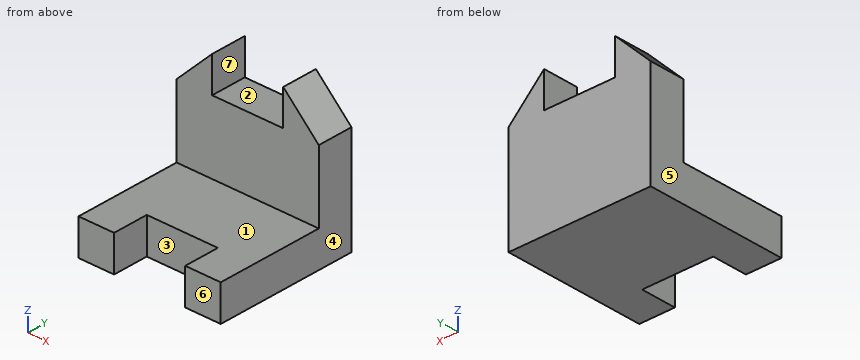
from build123d import *

# Parameters (mm, degrees)
F0_W      = 101.6
F0_H      = 101.6
F1_DEPTH  = 101.6
F2_W      = 50.8
F2_H      = 25.4
F3_DEPTH  = 25.4
F4_W      = 101.6
F4_H      = 76.2
F5_DEPTH  = 76.2
F7_DEPTH  = 25.4
F8_W      = 50.8
F8_H      = 50.8
F9_DEPTH  = 25.4
F9_FACE_W = 50.8
F9_FACE_H = 25.4
F10_DEPTH = 50.8
F11_W     = 50.8
F11_H     = 25.188574
F12_DEPTH = 59.436


with BuildPart() as f1:
    # F0 (on Front) → F1 (new body)
    with BuildSketch(Plane.XZ):
        with Locations((-5.817418, 8.951449)):
            Rectangle(F0_W, F0_H)
    extrude(amount=F1_DEPTH)

    # F2 (on face) → F3 (cut)
    with BuildSketch(Plane.XZ.offset(101.6)):
        with Locations((-5.817418, -29.148551)):
            Rectangle(F2_W, F2_H)
    extrude(amount=-F3_DEPTH, mode=Mode.SUBTRACT)

    # F4 (on face) → F5 (cut)
    with BuildSketch(Plane.XZ.offset(101.6)):
        with Locations((-5.817418, 21.651449)):
            Rectangle(F4_W, F4_H)
    extrude(amount=-F5_DEPTH, mode=Mode.SUBTRACT)

    # F6 (on face) → F7 (cut)
    with BuildSketch(Plane.XZ.offset(25.4)):
        Polygon((44.982582, 59.751449), (19.582582, 59.751449), (44.982582, 34.351449), align=None)
        Polygon((-31.217418, 59.751449), (-56.617418, 59.751449), (-56.617418, 34.351449), align=None)
    extrude(amount=-F7_DEPTH, mode=Mode.SUBTRACT)

    # F8 (on face) → F9 (cut)
    with BuildSketch(Plane.XZ.offset(25.4)):
        with Locations((-5.817418, 34.351449)):
            Rectangle(F8_W, F8_H)
    extrude(amount=-F9_DEPTH, mode=Mode.SUBTRACT)

    # F9_face (on face) → F10 (join)
    with BuildSketch(Plane(origin=(-5.817418, -12.7, 8.951449), x_dir=(1, 0, 0), z_dir=(0, 0, 1))):
        Rectangle(F9_FACE_W, F9_FACE_H)
    extrude(amount=F10_DEPTH)

    # F11 (on face) → F12 (cut)
    with BuildSketch(Plane.XZ.offset(25.4)):
        with Locations((-5.817418, 47.157162)):
            Rectangle(F11_W, F11_H)
    extrude(amount=-F12_DEPTH, mode=Mode.SUBTRACT)


solid = f1.part
Source: CAD feature listing. Evaluate the final solid. Frame: model axes, mm. Face numbers are marked on the shaded views. A direction names the side the tool comes from. Round coordinates to 2 decimals unless told otherwise and drop trailing zeros. Order: outer loops, then holes, each group sorted by start corner. A loop starts at its lowest first (then second) coordinate and runs counter-clockwise, first axis right, second up. Notation, with made-up numbers: (87.5, 52) - (106.5, 52) arc R22 ccw to (106.5, 84) - close; hole circle Ø6 at (66, 70). An arc over 180 degrees is marked (long way). Use a Markdown table: item, result. Add a question column.
1. Set-up query: the marked faces 1, 2 and 3. Return all of +Z, -Z, +X, -X, +Y, -Y with unobstructed straight access to the full face (end or side cutting, diameter ignored); none if empty.
2. Section query C-C (z = 52.5). Return the cut outline in (x, y).
3. Section query B-B (x = 10). Return the cut outline in (y, z), then the cut area to 3 significant figures.
4. Line query: probe 1 along X at (y, z) = (-86.5, -22); probe 2 along Y at (x, z) = (-19.5, 16.5); probe 3 along Z at (x, y) = (-18.5, -20.5). Output: solid intervals per line, ascending.
5. Mould query, pull axis X, two halves, no side actions, for the marked faces 4, 5, 6 and 7. Classes: +X half, -X half, draft (parallel to the pull), parting line (faces both ways), or undercut.
6. First-contact query: pin 1 (8 mm diameter, centred on x = -12.5, y = -71, fed in from +Z); pin 2 (20.5 mm diameter, centred on x = -8.5, y = -9, fed in from +Z); pin 3 (7.5 mm diameter, centred on y = -18, z = 46.5, fed in from +X). Flat tips, straight axial feed; report the tip coordinate or a pass-through.
7. Section query A-A (z = -27). Return the cut outline in (x, y), then the cut area to 3 significant figures.
8. Section query D-D (y = -46). Return the cut outline in (x, z).
Derived:
| question | item | result |
|---|---|---|
| 1 | face 1 | +Z, +X, -X, -Y |
| 1 | face 2 | +Z, +Y, -Y |
| 1 | face 3 | +Z, -Z, -Y |
| 2 | outline | (-38.47, -25.4) - (-31.22, -25.4) - (-31.22, 0) - (-38.47, 0) - close; (19.58, -25.4) - (26.83, -25.4) - (26.83, 0) - (19.58, 0) - close |
| 3 | outline | (-76.2, -41.85) - (0, -41.85) - (0, 34.56) - (-25.4, 34.56) - (-25.4, -16.45) - (-76.2, -16.45) - close |
| 3 | area | 3,230 mm2 |
| 4 | probe 1 | -56.62 to -31.22, 19.58 to 44.98 |
| 4 | probe 2 | -25.4 to 0 |
| 4 | probe 3 | -41.85 to 34.56 |
| 5 | face 4 | +X half |
| 5 | face 5 | -X half |
| 5 | face 6 | draft |
| 5 | face 7 | undercut |
| 6 | pin 1 | z = -16.45 |
| 6 | pin 2 | z = 34.56 |
| 6 | pin 3 | x = 36.58 |
| 7 | outline | (-56.62, -101.6) - (-31.22, -101.6) - (-31.22, -76.2) - (19.58, -76.2) - (19.58, -101.6) - (44.98, -101.6) - (44.98, 0) - (-56.62, 0) - close |
| 7 | area | 9,030 mm2 |
| 8 | outline | (-56.62, -41.85) - (44.98, -41.85) - (44.98, -16.45) - (-56.62, -16.45) - close |
